Geometry check sheet. Reference: the model listing, model coordinates, mm. A direction names the side the tool comes from. Give positions to 0.01 mm unless a question says otherwise; leave off trailing zeros. Order: outer loops, then holes, each group sorted by start corner. A loop starts at its lowest first (then second) coordinate and runs counter-clockwise, first axis right, second up.
```python
from build123d import *

# Parameters (mm, degrees)
F1_DEPTH  = 3.175
F2_W      = 177.8
F2_H      = 25.4
F3_DEPTH  = 25.4
F4_W      = 184.15
F4_H      = 25.4
F5_DEPTH  = 25.4
F7_R      = 3.175
F8_DEPTH  = 25.4
F9_W      = 133.35
F9_H      = 412.75
F10_DEPTH = 25.4
F11_W     = 50.8
F11_H     = 25.4
F12_DEPTH = 530.225
F13_W     = 50.8
F13_H     = 25.4
F14_DEPTH = 47.625


with BuildPart() as f1:
    # F0 (on Front) → F1 (new body)
    with BuildSketch(Plane.XZ):
        Polygon((241.3, -231.775), (241.3, 231.775), (57.15, 231.775), (57.15, -104.775), (-57.15, -104.775), (-57.15, 231.775), (-241.3, 231.775), (-241.3, 79.375), (-241.3, -104.775), (-241.3, -231.775), align=None)
        Polygon((-215.9, 73.025), (-209.55, 79.375), (-82.55, 79.375), (-82.55, -104.775), (-215.9, -104.775), align=None, mode=Mode.SUBTRACT)
        Polygon((82.55, -104.775), (82.55, 79.375), (209.55, 79.375), (215.9, 73.025), (215.9, -104.775), align=None, mode=Mode.SUBTRACT)
    extrude(amount=F1_DEPTH)

    # F2 (on face) → F3 (join)
    with BuildSketch(Plane.YZ.offset(241.3)):
        with Locations((-88.9, 117.475)):
            Rectangle(F2_W, F2_H)
    extrude(amount=-F3_DEPTH)

    # F4 (on face) → F5 (join)
    with BuildSketch(Plane.XZ.offset(177.8)):
        with Locations((149.225, 117.475)):
            Rectangle(F4_W, F4_H)
    extrude(amount=-F5_DEPTH)

    # F6: F1 across plane


with BuildPart() as f1_1:
    add(f1.part)
    add(f1.part.mirror(Plane.YZ))

    # F7 (on face) → F8 (cut)
    with BuildSketch(Plane.XZ.offset(3.175)):
        with Locations((-215.9, 79.375)):
            Circle(F7_R)
        with Locations((215.9, 79.375)):
            Circle(F7_R)
    extrude(amount=-F8_DEPTH, mode=Mode.SUBTRACT)

    # F9 (on face) → F10 (join)
    with BuildSketch(Plane(origin=(0, 0, 0), x_dir=(-1, 0, 0), z_dir=(0, 1, 0))):
        Polygon((-57.15, 231.775), (-241.3, 231.775), (-241.3, -206.375), (-241.3, -231.775), (241.3, -231.775), (241.3, 231.775), (57.15, 231.775), (57.15, -206.375), (-57.15, -206.375), align=None)
        with Locations((-149.225, 0)):
            Rectangle(F9_W, F9_H, mode=Mode.SUBTRACT)
        with Locations((149.225, 0)):
            Rectangle(F9_W, F9_H, mode=Mode.SUBTRACT)
    extrude(amount=F10_DEPTH)

    # F11 (on face) → F12 (join)
    with BuildSketch(Plane.YZ.offset(241.3)):
        with Locations((50.8, -136.525)):
            Rectangle(F11_W, F11_H)
    extrude(amount=-F12_DEPTH)

    # F13 (on face) → F14 (join)
    with BuildSketch(Plane.YZ.offset(241.3)):
        with Locations((50.8, -136.525)):
            Rectangle(F13_W, F13_H)
    extrude(amount=F14_DEPTH)


solid = f1_1.part
```
Q1. Cross-section at D-D, the plane x = 95. Record the boundary of the cut face in (y, z) (3 decimals), and give its area (3 significant figures).
Q2. Gauge pin test, flat ends, axial feed: P1, Ø4, axis at x = -221.5, y = -16.5, coming from the +Z side (3 decimals); P2, Ø20.5, axis at y = -72.5, z = 121.5, coming from the -X side; P3, Ø20.5, axis at x = 148.5, z = 122, coming from the +Y side. Record the tip position at first contact, or that the pin passes through.
Q3. Thickness scan on L1, parallel to Z at x = 215, y = -1 (3 decimals); L2, parallel to Y at x = -61, z = 86.5 (3 decimals); L3, parallel to Y at x = 41, z = -107.5 (3 decimals). Record the ranges inside material, lowest first.
Q4. Cross-section at B-B, the plane y = -106. Record the boundary of the cut face in (x, z) (3 decimals).
Q5. Release check for a two-part mould opening along X. For faces 1 (the face through (-265, 25.4, -137)), 2 (the face through (57.15, 11, 10)), 3 (the face through (-241.3, -1, 16)) record: pulls with the +X half, pulls with the -X half, needs draft (parallel to the pull), parting line crosses it, or undercut.
Q6. Cross-section at A-A, the plane z = 159. Record the boundary of the cut face in (x, y) (3 decimals).
Q7. Access from +Z, -Z, +X, -X, +Y, -Y to the whole of each face (thin tool, end or side, straight path). Record for faces 4 (the face through (218, 25.4, 81)), 5 (the face through (-57.15, -165, 117)), 6 (the face through (-4, 50, -149.225)), 7 (the face through (-148, 13, 206.375)), 8 (the face through (-148, 0, -156)).
Q8. Cross-section at C-C, the plane z = 61.5. Record the boundary of the cut face in (x, y) (3 decimals).
Answers follow:
1. outline: (-177.8, 104.775) - (-152.4, 104.775) - (-152.4, 130.175) - (-177.8, 130.175) - close; (-3.175, -231.775) - (25.4, -231.775) - (25.4, -206.375) - (0, -206.375) - (0, -104.775) - (-3.175, -104.775) - close; (-3.175, 79.375) - (0, 79.375) - (0, 206.375) - (25.4, 206.375) - (25.4, 231.775) - (-3.175, 231.775) - close; (25.4, -149.225) - (76.2, -149.225) - (76.2, -123.825) - (25.4, -123.825) - close
1. area: 4,110 mm2
2. P1: stops at z = 130.175
2. P2: stops at x = -241.3
2. P3: stops at y = 0
3. L1: z = -231.775 to -104.775, 73.925 to 76.33, 82.42 to 231.775
3. L2: y = -3.175 to 25.4
3. L3: y = -3.175 to 0
4. outline: (-241.3, 104.775) - (-215.9, 104.775) - (-215.9, 130.175) - (-241.3, 130.175) - close; (215.9, 104.775) - (241.3, 104.775) - (241.3, 130.175) - (215.9, 130.175) - close
5. face 1: needs draft
5. face 2: undercut
5. face 3: pulls with the -X half
6. outline: (-241.3, -3.175) - (-57.15, -3.175) - (-57.15, 25.4) - (-82.55, 25.4) - (-82.55, 0) - (-215.9, 0) - (-215.9, 25.4) - (-241.3, 25.4) - close; (57.15, -3.175) - (241.3, -3.175) - (241.3, 25.4) - (215.9, 25.4) - (215.9, 0) - (82.55, 0) - (82.55, 25.4) - (57.15, 25.4) - close
7. face 4: +Z, +X, -X, +Y
7. face 5: +Z, -Z, +Y, -Y
7. face 6: -Z, +X, -X, +Y
7. face 7: +Y
7. face 8: none
8. outline: (-241.3, -3.175) - (-215.9, -3.175) - (-215.9, 25.4) - (-241.3, 25.4) - close; (-82.55, -3.175) - (-57.15, -3.175) - (-57.15, 25.4) - (-82.55, 25.4) - close; (57.15, -3.175) - (82.55, -3.175) - (82.55, 25.4) - (57.15, 25.4) - close; (215.9, -3.175) - (241.3, -3.175) - (241.3, 25.4) - (215.9, 25.4) - close
